```python
from build123d import *

# Parameters (mm, degrees)
BOSS_EXTRUDE1_DEPTH                             = 6.35
SKETCH4_R                                       = 12.7
CUT_EXTRUDE3_DEPTH                              = 116.178567885
SKETCH5_R                                       = 15.875
CUT_EXTRUDE4_DEPTH                              = 4.5085
FILLET1_R                                       = 25.4
CUT_EXTRUDE5_DEPTH                              = 9.525
FILLET2_R                                       = 6.35
F_8_32_TAPPED_HOLE1_D                           = 3.4544
F_8_32_TAPPED_HOLE1_DEPTH                       = 10.668
F_8_32_TAPPED_HOLE1_TIP                         = 1.037806461
CSK_FOR_10_FLAT_HEAD_MACHINE_SCREW1_D           = 5.1054
CSK_FOR_10_FLAT_HEAD_MACHINE_SCREW1_CSINK_D     = 9.779
CSK_FOR_10_FLAT_HEAD_MACHINE_SCREW1_CSINK_ANGLE = 82


with BuildPart() as part:
    # Sketch1 → Boss-Extrude1 (new, symmetric)
    with BuildSketch(Plane.XY):
        with BuildLine():
            Line((25.4, 0), (25.4, -63.5))
            Line((25.4, -63.5), (-95.25, -63.5))
            Line((-95.25, -63.5), (-95.25, -31.75))
            Line((-95.25, -31.75), (-13.866905739, 21.280717216))
            ThreePointArc((-13.866905739, 21.280717216), (12.10249136, 22.33136142), (25.4, 0))
        make_face()
    extrude(amount=BOSS_EXTRUDE1_DEPTH, both=True)

    # Sketch4 → Cut-Extrude3 (cut, through all)
    with BuildSketch(Plane.XY.offset(6.35)):
        Circle(SKETCH4_R)
    extrude(amount=-CUT_EXTRUDE3_DEPTH, mode=Mode.SUBTRACT)

    # Sketch5 → Cut-Extrude4 (cut)
    with BuildSketch(Plane(origin=(0, 0, 6.35), x_dir=(-1, 0, 0), z_dir=(0, 0, -1))):
        Circle(SKETCH5_R)
    extrude(amount=CUT_EXTRUDE4_DEPTH, mode=Mode.SUBTRACT)

    # Fillet1
    fillet1_edges = [part.edges().sort_by_distance(p)[0] for p in [
        (-95.25, -31.75, 0),
    ]]
    fillet(fillet1_edges, radius=FILLET1_R)

    # Sketch9 → Cut-Extrude5 (cut)
    with BuildSketch(Plane.XY.offset(6.35)):
        with BuildLine():
            Line((-10.400179304, 15.960537912), (-80.250179304, -29.555003506))
            ThreePointArc((-80.250179304, -29.555003506), (-86.598521065, -36.438672898), (-88.9, -45.515541418))
            Line((-88.9, -45.515541418), (-88.9, -57.15))
            Line((-88.9, -57.15), (19.05, -57.15))
            Line((19.05, -57.15), (19.05, 0))
            ThreePointArc((19.05, 0), (-9.07686852, -16.748521065), (-10.400179304, 15.960537912))
        make_face()
    extrude(amount=-CUT_EXTRUDE5_DEPTH, mode=Mode.SUBTRACT)

    # Fillet2
    fillet2_edges = [part.edges().sort_by_distance(p)[0] for p in [
        (-10.400179304, 15.960537912, 1.5875),
        (19.05, 0, 1.5875),
        (19.05, -57.15, 1.5875),
        (-88.9, -57.15, 1.5875),
    ]]
    fillet(fillet2_edges, radius=FILLET2_R)

    # #8-32 Tapped Hole1
    with Locations(Plane.XZ.offset(63.5)):
        with Locations((-82.55, 0), (-34.925, 0), (12.7, 0)):
            Hole(F_8_32_TAPPED_HOLE1_D / 2, depth=F_8_32_TAPPED_HOLE1_DEPTH)
            with Locations((0, 0, -(F_8_32_TAPPED_HOLE1_DEPTH + F_8_32_TAPPED_HOLE1_TIP / 2))):  # 118° drill point
                Cone(0, F_8_32_TAPPED_HOLE1_D / 2, F_8_32_TAPPED_HOLE1_TIP, mode=Mode.SUBTRACT)

    # CSK for #10 Flat Head Machine Screw1 (through all)
    with Locations(Plane(origin=(0, 0, -6.35), x_dir=(-1, 0, 0), z_dir=(0, 0, -1))):
        with Locations((44.45, -25.4)):
            CounterSinkHole(CSK_FOR_10_FLAT_HEAD_MACHINE_SCREW1_D / 2, CSK_FOR_10_FLAT_HEAD_MACHINE_SCREW1_CSINK_D / 2, counter_sink_angle=CSK_FOR_10_FLAT_HEAD_MACHINE_SCREW1_CSINK_ANGLE)


solid = part.part
```
Design review of the part built by this model. Coordinates are the model's own, in mm. A direction names the side the tool comes from. Coordinates: 2 decimals unless noted, no trailing zeros. Write each loop counter-clockwise with the first axis right and the second up, starting at its lowest first coordinate (ties: lowest second). Pieces come first, ordered by that corner, then holes. Notation, with made-up numbers: M -34.75,-7 L -17.75,-7 A5 cw -17.75,2 Z; hole C 69.25,58.5 d1. An arc over 180 degrees is marked long. Answer as a JSON object with one key per item and string values.
Item 1: Add section B-B, the plane z = 0. Give the boundary of the cut face in (x, y) (3 decimals), and give its area (3 significant figures).
Outcome:
{"outline": "M -95.25,-63.5 L -84.277,-63.5 L -84.277,-56.911 A6.35 cw -88.9,-50.8 L -88.9,-45.516 A19.05 cw -80.25,-29.555 L -28.83,3.951 A6.35 cw -19.022,-1.027 A19.05 ccw 9.525,-16.498 A6.35 cw 19.05,-21.997 L 19.05,-50.8 A6.35 cw 14.427,-56.911 L 14.427,-63.5 L 25.4,-63.5 L 25.4,0 A25.4 ccw -13.867,21.281 L -83.717,-24.235 A25.4 ccw -95.25,-45.516 Z; M -80.823,-63.5 L -36.652,-63.5 L -36.652,-57.15 L -80.823,-57.15 Z; M -33.198,-63.5 L 10.973,-63.5 L 10.973,-57.15 L -33.198,-57.15 Z; hole C 0,0 d25.4", "area": "2,850 mm²"}
Item 2: Add section C-C, the plane x = -74. Give the boundary of the cut face in (y, z) (3 decimals), and give its area (3 significant figures).
Outcome:
{"outline": "M -63.5,-6.35 L -17.903,-6.35 L -17.903,6.35 L -25.482,6.35 L -25.482,-3.175 L -57.15,-3.175 L -57.15,6.35 L -63.5,6.35 Z", "area": "277 mm²"}
Item 3: Wall thickness on probe 1 along Y at (x, z) = (0, 4.3) (3 decimals); probe 2 along X at (y, z) = (3, 4.25); probe 3 along X at (y, z) = (-2, -0.75): over which ranges is each line inside the solid? List them lowest first.
Outcome:
{"probe 1": "-63.5 to -57.15, -19.05 to -15.875, 15.875 to 25.4", "probe 2": "-41.92 to -30.29, -20.75 to -15.59, 15.59 to 25.22", "probe 3": "-49.59 to -37.96, -18.94 to -12.54, 12.54 to 25.4"}
Item 4: Machinability: for faces 1 (the cylindrical face through (-86.535, -36.322, 1.654)), 2 (the flat face through (-49.281, -1.796, 0.089)), which of the approach directions +Z, -Z, +X, -X, +Y, -Y give a long, thin tool a straight path to every point of the face, cutting with its end or side? Answer none if there is none.
Outcome:
{"face 1": "+Z", "face 2": "+Z, -Z, -X, +Y"}
Item 5: Insertion check: pin 1 Ø3 at (x, z) = (-34.925, 0) entering from +Y; pin 2 Ø3 at (x, z) = (-82.55, 0) entering from -Y; pin 3 Ø6 at (y, z) = (-3.5, -2) entering from -X. Each pin has a flat end and moves straight along its axis. Give the tip position at first contact, or say it passes through.
Outcome:
{"pin 1": "y = 8.54", "pin 2": "y = -32.82", "pin 3": "x = -56.5"}
Item 6: Draft analysis for pull direction Z (two halves, no side actions). For faces 3 (the flat face through (-21, -28, -6.35)), 4 (the flat face through (-36, -57.15, 2)), 5 (the cylindrical face through (-33.652, -60.281, 1.167)), state which applies: pulls with the +Z half, pulls with the -Z half, needs draft (parallel to the pull), parting line crosses it, or undercut.
Outcome:
{"face 3": "pulls with the -Z half", "face 4": "needs draft", "face 5": "undercut"}
